from build123d import *

# Parameters (mm, degrees)
CROQUIS1_R              = 25
CROQUIS1_R_2            = 11
SALIENTE_EXTRUIR1_DEPTH = 5
CROQUIS2_R              = 2.5
CORTAR_EXTRUIR1_DEPTH   = 10


with BuildPart() as part:
    # Croquis1 → Saliente-Extruir1 (new body)
    with BuildSketch(Plane(origin=(0, 0, 0), x_dir=(0, 0, -1), z_dir=(1, 0, 0))):
        Circle(CROQUIS1_R)
        Circle(CROQUIS1_R_2, mode=Mode.SUBTRACT)
    extrude(amount=SALIENTE_EXTRUIR1_DEPTH)

    # Croquis2 → Cortar-Extruir1 (cut)
    with BuildSketch(Plane(origin=(5, 0, 0), x_dir=(0, 0, -1), z_dir=(1, 0, 0))):
        with Locations((0, 21)):
            Circle(CROQUIS2_R)
        with Locations((21, 0)):
            Circle(CROQUIS2_R)
        with Locations((0, -21)):
            Circle(CROQUIS2_R)
        with Locations((-21, 0)):
            Circle(CROQUIS2_R)
    extrude(amount=-CORTAR_EXTRUIR1_DEPTH, mode=Mode.SUBTRACT)


solid = part.part
Geometry: final body of the model. Coordinates: model frame, mm. Round coordinates to 2 decimals unless told otherwise and drop trailing zeros. Loops run counter-clockwise (first coordinate to the right, second up) from the corner with the lowest first, then second, coordinate; pieces in that order, holes last.
Q1. Section D-D on y = -21. Return loops of the section in (x, z), plus the area to 3 significant figures.
Q2. Pin query (flat end, axial travel): P1, Ø2, axis at x = 3.5, z = 5, coming from the -Y side; P2, Ø1, axis at x = 1.5, z = 13.5, coming from the -Y side; P3, Ø1, axis at x = 3.5, z = 19.5, coming from the +Y side. Return the tip coordinate at first contact, or that it passes through.
Q3. Section A-A on z = 0. Return loops of the section in (x, y).
Q4. Pull-direction query (Z, two-part tool) for faces 1 (the flat face through (5, -11, -5)), 2 (the cylindrical face through (2.465, 7.509, -23.846)), 3 (the cylindrical face through (2.54, 23.48, 0.33)); classes: released by +Z, released by -Z, zero draft, split by the parting line, or undercut.
Q5. Material intervals for L1, parallel to Y at x = 3.2, z = 0; L2, parallel to Z at x = 1.5, y = -1.5; L3, parallel to Z at x = 1.15, y = 8, sorted ascending.
Q6. Section C-C on x = 0.75. Return loops of the section in (y, z), plus the area to 3 significant figures.
Evaluation:
1. outline: (0, -13.56) - (5, -13.56) - (5, -2.5) - (0, -2.5) - close; (0, 2.5) - (5, 2.5) - (5, 13.56) - (0, 13.56) - close
1. area: 111 mm2
2. P1: stops at y = -24.68
2. P2: stops at y = -21.35
2. P3: stops at y = 16.25
3. outline: (0, -25) - (5, -25) - (5, -23.5) - (0, -23.5) - close; (0, -18.5) - (5, -18.5) - (5, -11) - (0, -11) - close; (0, 11) - (5, 11) - (5, 18.5) - (0, 18.5) - close; (0, 23.5) - (5, 23.5) - (5, 25) - (0, 25) - close
4. face 1: zero draft
4. face 2: split by the parting line
4. face 3: undercut
5. L1: y = -25 to -23.5, -18.5 to -11, 11 to 18.5, 23.5 to 25
5. L2: z = -24.95 to -23, -19 to -10.9, 10.9 to 19, 23 to 24.95
5. L3: z = -23.69 to -7.55, 7.55 to 23.69
6. outline: circle Ø50 at (0, 0); hole circle Ø5 at (-21, 0); hole circle Ø22 at (0, 0); hole circle Ø5 at (0, -21); hole circle Ø5 at (0, 21); hole circle Ø5 at (21, 0)
6. area: 1,500 mm2
